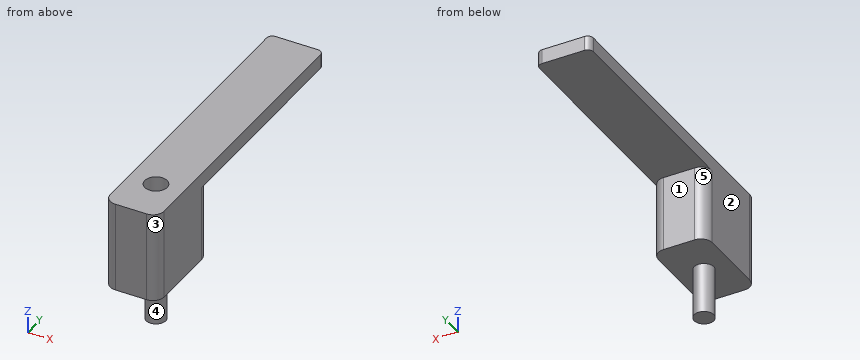
Autodesk Inventor part; units mm, degrees
ref_plane "YZ Plane" through (0, 0, 0) normal (1, 0, 0) x (0, 1, 0)
ref_plane "XZ Plane" through (0, 0, 0) normal (0, 1, 0) x (-1, 0, 0)
ref_plane "XY Plane" through (0, 0, 0) normal (0, 0, 1) x (1, 0, 0)
sketch "Sketch8" plane through (0, 0, 0) normal (0, 0, 1) x (1, 0, 0)
  line L0 (0, 0) -> (-9.6, 0)
  line L1 (-9.6, 0) -> (-9.6, 53)
  line L2 (-9.6, 53) -> (0, 53)
  line L3 (0, 53) -> (0, 0)
  line L4 (0, 4) -> (-9.6, 4)
  line L5 (-4.8, 4) -> (-4.8, 12)
  circle A0 centre (-4.8, 8) radius 2
  point P0 (-4.8, 6)
  point P1 (-4.8, 10)
  dimension "d23" = 9.6
  dimension "d24" = 53
  dimension "d25" = 8
  dimension "d26" = 4
extrude "Extrusion7" add sketch "Sketch8" along normal blind 2.6
sketch "Sketch9" plane through (0, 0, 0) normal (0, 0, -1) x (-1, 0, 0)
  line L0 (0, 0) -> (9.6, 0)
  line L1 (9.6, 0) -> (9.6, 16)
  line L2 (9.6, 16) -> (0, 16)
  line L3 (0, 16) -> (0, 0)
  dimension "d29" = 9.6
  dimension "d30" = 16
extrude "Extrusion8" add sketch "Sketch9" along normal blind 13.5
sketch "Sketch10" plane through (0, 0, -13.5) normal (0, 0, -1) x (-1, 0, 0)
  circle A0 centre (4.8, 8) radius 1.75
  circle A1 centre (4.8, 8) radius 1.75
  point P0 (0, 0)
  dimension "d33" = 3.5
  dimension "d41" = 3.5
extrude "Extrusion9" add sketch "Sketch10" along normal blind 9
fillet "Fillet2" radius 2 4 edges at (-9.6, 16, -6.75) (0, 16, -6.75) (-9.6, 0, -5.45) (0, 0, -5.45)
fillet "Fillet3" radius 1 2 edges at (-9.6, 53, 1.3) (0, 53, 1.3)
sketch "Sketch11" plane through (-4.8, 8, 0) normal (0, 0, 1) x (1, 0, 0)
  circle A0 centre (0, 0) radius 2
  point P0 (4.8, -8)
  dimension "d38" = 4
extrude "Extrusion10" cut sketch "Sketch11" against normal blind 10
properties part number "Hook_TestFit"
The listing builds one solid part. Answer for the finished solid, in the listing's coordinates (mm). Face numbers are marked on the shaded views. A direction names the side the tool comes from. Coordinates: 2 decimals unless noted, no trailing zeros. Loops run counter-clockwise (first coordinate to the right, second up) from the corner with the lowest first, then second, coordinate; pieces in that order, holes last. Notation, with made-up numbers: M 82.25,-25.5 L 117.25,-25.5 A17 cw 117.25,5.5 Z; hole C 5,-40 d11. An arc over 180 degrees is marked long. Answer in a Markdown table with one row per item.
1) Find section C-C (y = 8). Determine the outline of the cut face in (x, z).
Answers below:
| item | result |
|---|---|
| outline | M -9.6,-13.5 L -6.55,-13.5 L -6.55,-22.5 L -3.05,-22.5 L -3.05,-13.5 L 0,-13.5 L 0,2.6 L -2.8,2.6 L -2.8,-10 L -6.8,-10 L -6.8,2.6 L -9.6,2.6 Z |
2) Find section A-A (z = -3.25). Determine the outline of the cut face in (x, y).
Answers below:
| item | result |
|---|---|
| outline | M -9.6,2 A2 ccw -7.6,0 L -2,0 A2 ccw 0,2 L 0,14 A2 ccw -2,16 L -7.6,16 A2 ccw -9.6,14 Z; hole C -4.8,8 d4 |
3) Find section D-D (z = -15.5). Determine the outline of the cut face in (x, y).
Answers below:
| item | result |
|---|---|
| outline | C -4.8,8 d3.5 |
4) Find section B-B (x = -4.8). Determine the outline of the cut face in (y, z), then the cut area to 3 significant figures.
Answers below:
| item | result |
|---|---|
| outline | M 0,-13.5 L 6.25,-13.5 L 6.25,-22.5 L 9.75,-22.5 L 9.75,-13.5 L 16,-13.5 L 16,0 L 53,0 L 53,2.6 L 10,2.6 L 10,-10 L 6,-10 L 6,2.6 L 0,2.6 Z |
| area | 335 mm^2 |
5) Find the intervals of material crossed by probe 1 along X at (y, z) = (8, -3.75); probe 2 along Y at (x, z) = (-4.8, -3); probe 3 along Z at (x, y) = (-3, 10), in increasing order.
Answers below:
| item | result |
|---|---|
| probe 1 | -9.6 to -6.8, -2.8 to 0 |
| probe 2 | 0 to 6, 10 to 16 |
| probe 3 | -13.5 to 2.6 |
6) Which of the six approach directions +Z, -Z, +X, -X, +Y, -Y give full straight-line access (tool end or side, diameter ignored) to the marked faces 1, 2, 3, 4 and 5?
Answers below:
| item | result |
|---|---|
| face 1 | -Z, +X, -X, +Y |
| face 2 | +Z, -Z, -X, +Y, -Y |
| face 3 | +Z, -Z, +X, -Y |
| face 4 | -Z |
| face 5 | -Z, -X, +Y |
7) Given pin 1 (1 mm diameter, centred on x = -2.5, y = 5.5, fed in from -Z); pin 2 (3 mm diameter, centred on x = -5.5, z = -8.5, fed in from +Y); pin 3 (5 mm diameter, centred on x = -5.5, y = 41, fed in from -Z); pin 4 (1.5 mm diameter, centred on y = 26.5, z = -1, fed in from -X), each flat-ended and moving along its own axis, determine where each tip first touches the part or whether it passes through.
Answers below:
| item | result |
|---|---|
| pin 1 | z = -13.5 |
| pin 2 | y = 16 |
| pin 3 | z = 0 |
| pin 4 | through |
